Here's how the part is built. I have some questions about the finished solid (model axes, mm). A direction names the side the tool comes from. Give positions to 0.01 mm unless a question says otherwise; leave off trailing zeros. Write each loop counter-clockwise with the first axis right and the second up, starting at its lowest first coordinate (ties: lowest second). Pieces come first, ordered by that corner, then holes. Notation, with made-up numbers: (-35, -33.75) - (-11, -33.75) arc R15 ccw to (-11, -9.75) - close; hole circle Ø11 at (-20, 61.5). An arc over 180 degrees is marked (long way). Use a Markdown table: item, result.
```python
from build123d import *

# Parameters (mm, degrees)
SKETCH1_W           = 45
SKETCH1_H           = 20
SKETCH1_R           = 4.6
SKETCH1_W_2         = 20
SKETCH1_H_2         = 14
SKETCH1_R_2         = 2.5
BOSS_EXTRUDE1_DEPTH = 4
BOSS_EXTRUDE2_START = 4
SKETCH1_4_W         = 20
SKETCH1_4_H         = 14
BOSS_EXTRUDE2_DEPTH = 20
CUT_EXTRUDE1_START  = 4
SKETCH1_5_R         = 4.6
CUT_EXTRUDE1_DEPTH  = 2.2
CUT_EXTRUDE2_START  = -20
SKETCH2_R           = 4.6
CUT_EXTRUDE2_DEPTH  = 16
SKETCH2_6_R         = 2.525
CUT_EXTRUDE3_DEPTH  = 4
SKETCH2_7_R         = 4.45
SKETCH2_7_R_2       = 2.525
CUT_EXTRUDE4_DEPTH  = 1.5
FILLET1_R           = 3
CHAMFER1_SIZE       = 2.25


with BuildPart() as part:
    # Sketch1 → Boss-Extrude1 (new body)
    # profile 1 of 4: a face of its own
    with BuildSketch(Plane(origin=(0, 0, 0), x_dir=(1, 0, 0), z_dir=(0, 1, 0))):
        Rectangle(SKETCH1_W, SKETCH1_H)
        with Locations((15, 0)):
            Circle(SKETCH1_R, mode=Mode.SUBTRACT)
        with Locations((-15, 0)):
            Circle(SKETCH1_R, mode=Mode.SUBTRACT)
        Rectangle(SKETCH1_W_2, SKETCH1_H_2, mode=Mode.SUBTRACT)
    # profile 2 of 4: a face of its own
    with BuildSketch(Plane(origin=(0, 0, 0), x_dir=(1, 0, 0), z_dir=(0, 1, 0))):
        with Locations((-15, 0)):
            Circle(SKETCH1_R)
        with Locations(Location((-15, 0, 0), (0, 0, 270))):
            Circle(SKETCH1_R_2, mode=Mode.SUBTRACT)
    # profile 3 of 4: a face of its own
    with BuildSketch(Plane(origin=(0, 0, 0), x_dir=(1, 0, 0), z_dir=(0, 1, 0))):
        with Locations((15, 0)):
            Circle(SKETCH1_R)
        with Locations(Location((15, 0, 0), (0, 0, 270))):
            Circle(SKETCH1_R_2, mode=Mode.SUBTRACT)
    # profile 4 of 4: a face of its own
    with BuildSketch(Plane(origin=(0, 0, 0), x_dir=(1, 0, 0), z_dir=(0, 1, 0))):
        Rectangle(SKETCH1_W_2, SKETCH1_H_2)
    extrude(amount=BOSS_EXTRUDE1_DEPTH)

    # Sketch1<4> → Boss-Extrude2 (add)
    with BuildSketch(Plane(origin=(0, 0, 0), x_dir=(1, 0, 0), z_dir=(0, 1, 0)).offset(BOSS_EXTRUDE2_START)):
        Rectangle(SKETCH1_4_W, SKETCH1_4_H)
    extrude(amount=BOSS_EXTRUDE2_DEPTH)

    # Sketch1<5> → Cut-Extrude1 (cut)
    with BuildSketch(Plane(origin=(0, 0, 0), x_dir=(1, 0, 0), z_dir=(0, 1, 0)).offset(CUT_EXTRUDE1_START)):
        with Locations(Location((15, 0, 0), (0, 0, 270))):
            Circle(SKETCH1_5_R)
        with Locations(Location((-15, 0, 0), (0, 0, 270))):
            Circle(SKETCH1_5_R)
    extrude(amount=-CUT_EXTRUDE1_DEPTH, mode=Mode.SUBTRACT)

    # Sketch2 → Cut-Extrude2 (cut)
    with BuildSketch(Plane(origin=(10, 0, 0), x_dir=(0, 0, -1), z_dir=(1, 0, 0)).offset(CUT_EXTRUDE2_START)):
        with Locations(Location((0, 18, 0), (0, 0, 180))):
            Circle(SKETCH2_R)
    extrude(amount=CUT_EXTRUDE2_DEPTH, mode=Mode.SUBTRACT)

    # Sketch2<6> → Cut-Extrude3 (cut)
    with BuildSketch(Plane(origin=(10, 0, 0), x_dir=(0, 0, -1), z_dir=(1, 0, 0))):
        with Locations((0, 18)):
            Circle(SKETCH2_6_R)
    extrude(amount=-CUT_EXTRUDE3_DEPTH, mode=Mode.SUBTRACT)

    # Sketch2<7> → Cut-Extrude4 (cut)
    with BuildSketch(Plane(origin=(10, 0, 0), x_dir=(0, 0, -1), z_dir=(1, 0, 0))):
        with Locations((0, 18)):
            Circle(SKETCH2_7_R)
        with Locations((0, 18)):
            Circle(SKETCH2_7_R_2, mode=Mode.SUBTRACT)
    extrude(amount=-CUT_EXTRUDE4_DEPTH, mode=Mode.SUBTRACT)

    # Fillet1
    fillet1_edges = [part.edges().sort_by_distance(p)[0] for p in [
        (0, 4, 7),
        (0, 4, -7),
    ]]
    fillet(fillet1_edges, radius=FILLET1_R - 0.0001)  # a hair under: the kernel refuses the full size

    # Chamfer1
    chamfer1_edges = [part.edges().sort_by_distance(p)[0] for p in [
        (0, 24, -7),
        (0, 24, 7),
    ]]
    chamfer(chamfer1_edges, length=CHAMFER1_SIZE)


solid = part.part
```
Item 1: Will these pins go through, and if not, where does the flat tip stop? pin 1 Ø4 at (y, z) = (18, 0) entering from +X; pin 2 Ø6 at (y, z) = (8.5, -0.5) entering from -X; pin 3 Ø4 at (y, z) = (17.5, 2.5) entering from -X; pin 4 Ø10 at (y, z) = (18.5, 1.5) entering from +X.
Values:
| item | result |
|---|---|
| pin 1 | passes through |
| pin 2 | stops at x = -10 |
| pin 3 | stops at x = 6 |
| pin 4 | stops at x = 10 |
Item 2: I need wall thicknesses on line 1 along X through (y, z) = (1, 0); line 2 along X through (y, z) = (2.6, 0); line 3 along Y through (x, z) = (7.05, 0) (3 decimals). Which ranges of each line are inside material? Lowest first, please. Write a range as [from, to].
Values:
| item | result |
|---|---|
| line 1 | x = [-22.5, -17.5], [-12.5, 12.5], [17.5, 22.5] |
| line 2 | x = [-22.5, -19.6], [-10.4, 10.4], [19.6, 22.5] |
| line 3 | y = [0, 15.475], [20.525, 24] |
Item 3: Thinking about a two-plate mould opening in Y: for faces 5 (the flat face through (6, 20, 2)), 6 (the flat face through (13, 1.8, 2)), 7 (the flat face through (8.5, 16, -2)), 8 (the flat face through (0, 2, -10)), which applies, +Y half, -Y half, draft (parallel to the pull), parting line (faces both ways), or undercut?
Values:
| item | result |
|---|---|
| face 5 | undercut |
| face 6 | +Y half |
| face 7 | undercut |
| face 8 | draft |
Item 4: If we section it at A-A, the plane y = 18: Write out the boundary of the cut face in (x, z) (3 decimals).
Values:
| item | result |
|---|---|
| outline | (-10, -7) - (10, -7) - (10, -4.45) - (8.5, -4.45) - (8.5, -2.525) - (6, -2.525) - (6, -4.6) - (-10, -4.6) - close; (-10, 4.6) - (6, 4.6) - (6, 2.525) - (8.5, 2.525) - (8.5, 4.45) - (10, 4.45) - (10, 7) - (-10, 7) - close |
Item 5: If we section it at B-B, the plane x = 15: Write out the boundary of the cut face in (y, z).
Values:
| item | result |
|---|---|
| outline | (0, -10) - (4, -10) - (4, -4.6) - (1.8, -4.6) - (1.8, -2.5) - (0, -2.5) - close; (0, 2.5) - (1.8, 2.5) - (1.8, 4.6) - (4, 4.6) - (4, 10) - (0, 10) - close |
Item 6: If we section it at C-C, the plane z = 0: Count the separate pieces of the cut face and the enclosed holes in it, plus the area to 3 significant figures.
Values:
| item | result |
|---|---|
| separate pieces | 4 |
| enclosed holes | 0 |
| area | 348 mm2 |
Item 7: If we section it at D-D, the plane x = -12: Write out the boundary of the cut face in (y, z), plus the area to 3 significant figures.
Values:
| item | result |
|---|---|
| outline | (0, -10) - (4, -10) - (4, -3.49) - (1.8, -3.49) - (1.8, 3.49) - (4, 3.49) - (4, 10) - (0, 10) - close |
| area | 64.7 mm2 |
Item 8: For faces 1 (the flat face through (0, 14, -7)), 2 (the flat face through (-22.5, 2, 0)), 3 (the flat face through (-17, 1.8, 2)), 4 (the flat face through (-10, 12, 0)), which set-ups out of +Z, -Z, +X, -X, +Y, -Y let a thin tool reach every point of the face, with its end or its side?
Values:
| item | result |
|---|---|
| face 1 | -Z, +X, -X, +Y |
| face 2 | +Z, -Z, -X, +Y, -Y |
| face 3 | +Y |
| face 4 | +Z, -Z, -X, +Y |
